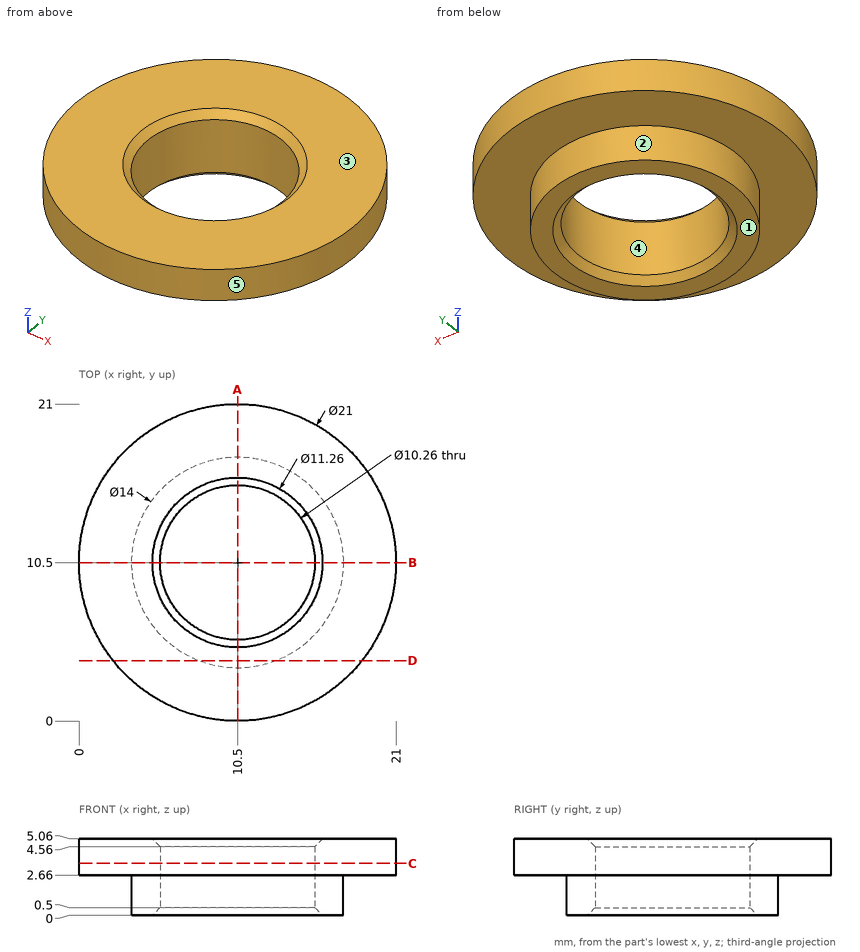
Verification items for this drawing (mm, ordinates from the low corner). A direction names the side the tool comes from. Give positions to 0.01 mm unless a question says otherwise; leave off trailing zeros. Loops run counter-clockwise (first coordinate to the right, second up) from the corner with the lowest first, then second, coordinate; pieces in that order, holes last. Notation, with made-up numbers: M 19.25,54.5 L 27.25,54.5 A8 ccw 27.25,61.5 Z; hole C -38.75,-34.5 d9. An arc over 180 degrees is marked long. Answer as a JSON object with one key per item and string values. Group by question number.
Q1. Cross-section at A-A on x = 10.5. Record the cut outline in (y, z).
Q2. Release check for a two-part mould opening along Y. For the marked faces 3, 4 and 5 record: released by +Y, released by -Y, zero draft, split by the parting line, or undercut.
Q3. Cross-section at C-C on z = 3.45. Record the cut outline in (x, y), then the cut area to 3 significant figures.
Q4. Go/stop test with flat-tipped pins: P1, Ø2, axis at x = 15, z = 4, coming from the +Y side; P2, Ø1, axis at x = 13, y = 2.5, coming from the -Z side. Record where each tip stops, or that it passes through.
Q5. Access from +Z, -Z, +X, -X, +Y, -Y to the whole of each face (thin tool, end or side, straight path). Record for the marked faces 1 and 2.
Q6. Material ranges on line 1 along Y through (x, z) = (10.5, 3.4); line 2 along Y through (x, z) = (10.5, 2.1); line 3 along Z through (x, y) = (7.25, 17.5), recorded low to high. Write a range as [from, to].
Q7. Cross-section at D-D on y = 4. Record the cut outline in (x, z), then the cut area to 3 significant figures.
Evaluation:
{
 "1": {"outline": "M 0,2.66 L 3.5,2.66 L 3.5,0 L 4.87,0 L 5.37,0.5 L 5.37,4.56 L 4.87,5.06 L 0,5.06 Z; M 15.63,0.5 L 16.13,0 L 17.5,0 L 17.5,2.66 L 21,2.66 L 21,5.06 L 16.13,5.06 L 15.63,4.56 Z"},
 "2": {"face 3": "zero draft", "face 4": "undercut", "face 5": "split by the parting line"},
 "3": {"outline": "C 10.5,10.5 d21; hole C 10.5,10.5 d10.26", "area": "264 mm2"},
 "4": {"P1": "stops at y = 20.4", "P2": "stops at z = 2.66"},
 "5": {"face 1": "-Z, +X, -X, +Y, -Y", "face 2": "-Z"},
 "6": {"line 1": "y = [0, 5.37], [15.63, 21]", "line 2": "y = [3.5, 5.37], [15.63, 17.5]", "line 3": "z = [2.66, 5.06]"},
 "7": {"outline": "M 2.25,2.66 L 7.9,2.66 L 7.9,0 L 13.1,0 L 13.1,2.66 L 18.75,2.66 L 18.75,5.06 L 2.25,5.06 Z", "area": "53.4 mm2"}
}
